Verification items for the finished model (mm, model axes). Round coordinates to 2 decimals unless told otherwise and drop trailing zeros. Order: outer loops, then holes, each group sorted by start corner. A loop starts at its lowest first (then second) coordinate and runs counter-clockwise, first axis right, second up. Notation, with made-up numbers: M 27,16.25 L 57,16.25 A19 ccw 57,31.25 Z; hole C 71,-25.5 d2. An arc over 180 degrees is marked long. Use one line per item in the form item = value. Start each with the question number.
Item 1: Go/stop test with flat-tipped pins: pin 1 Ø1.5 at (y, z) = (21, 1.5) entering from -X; pin 2 Ø3 at (y, z) = (-32.5, 1) entering from +X. Record where each tip stops, or that it passes through.
Item 2: Cross-section at A-A on x = 31.5. Enter the section's corners in (y, z).
Item 3: Cross-section at B-B on y = 22. Enter the section's corners in (x, z), then the cut area to 3 significant figures.
Item 4: Thickness scan on probe 1 along X at (y, z) = (-24, 4.75); probe 2 along X at (y, z) = (12.5, 1.8); probe 3 along Y at (x, z) = (-186, 1.5). Record the ranges inside material, lowest first. Write a range as [from, to].
Item 5: Cross-section at C-C on z = 2.9. Count the separate pieces of the cut face and the enclosed holes in it, then the cut area to 3 significant figures.
from build123d import *

# Parameters (mm, degrees)
SKETCH1_W           = 452
SKETCH1_H           = 90
BOSS_EXTRUDE1_DEPTH = 5
SKETCH2_W           = 5.2
SKETCH2_H           = 25.2
CUT_EXTRUDE1_DEPTH  = 231.490780727
SKETCH4_W           = 5
SKETCH4_H           = 30
CUT_EXTRUDE5_DEPTH  = 5
SKETCH7_R           = 1
CUT_EXTRUDE6_DEPTH  = 231.490780727
FILLET4_R           = 1
SKETCH8_W           = 20.2
SKETCH8_H           = 10
CUT_EXTRUDE7_DEPTH  = 10
SKETCH9_W           = 20.2
SKETCH9_H           = 10
CUT_EXTRUDE8_DEPTH  = 300


with BuildPart() as part:
    # Sketch1 → Boss-Extrude1 (new body)
    with BuildSketch(Plane.XY):
        Rectangle(SKETCH1_W, SKETCH1_H)
    extrude(amount=BOSS_EXTRUDE1_DEPTH)

    # Sketch2 → Cut-Extrude1 (cut, through all)
    with BuildSketch(Plane.XY.offset(5)):
        with Locations((0, 17.4)):
            Rectangle(SKETCH2_W, SKETCH2_H)
        with Locations((0, -17.4)):
            Rectangle(SKETCH2_W, SKETCH2_H)
    extrude(amount=-CUT_EXTRUDE1_DEPTH, mode=Mode.SUBTRACT)

    # Sketch4 → Cut-Extrude5 (cut)
    with BuildSketch(Plane.ZY.offset(226)):
        with Locations((2.5, 25)):
            Rectangle(SKETCH4_W, SKETCH4_H)
        with Locations((2.5, -25)):
            Rectangle(SKETCH4_W, SKETCH4_H)
    cut_extrude5 = extrude(amount=-CUT_EXTRUDE5_DEPTH, mode=Mode.SUBTRACT)

    # Mirror2: Cut-Extrude5 across plane
    add(cut_extrude5.mirror(Plane(origin=(0, 0, 0), x_dir=(0, 0, 1), z_dir=(1, 0, 0))), mode=Mode.SUBTRACT)

    # Sketch7 → Cut-Extrude6 (cut, through all)
    with BuildSketch(Plane.XY.offset(5)):
        with Locations((-221, 39)):
            Circle(SKETCH7_R)
        with Locations((-221, 11)):
            Circle(SKETCH7_R)
        with Locations((-221, -11)):
            Circle(SKETCH7_R)
        with Locations((-221, -39)):
            Circle(SKETCH7_R)
        with Locations((221, -39)):
            Circle(SKETCH7_R)
        with Locations((221, -11)):
            Circle(SKETCH7_R)
        with Locations((221, 11)):
            Circle(SKETCH7_R)
        with Locations((221, 39)):
            Circle(SKETCH7_R)
    extrude(amount=-CUT_EXTRUDE6_DEPTH, mode=Mode.SUBTRACT)

    # Fillet4
    fillet4_edges = [part.edges().sort_by_distance(p)[0] for p in [
        (221, 38, 2.5),
        (221, 12, 2.5),
        (221, -12, 2.5),
        (221, -38, 2.5),
        (-221, 38, 2.5),
        (-221, 12, 2.5),
        (-221, -38, 2.5),
        (-221, -12, 2.5),
        (-226, 10, 2.5),
        (-226, 40, 2.5),
        (-226, -40, 2.5),
        (-226, -10, 2.5),
        (226, 10, 2.5),
        (226, 40, 2.5),
        (226, -40, 2.5),
        (226, -10, 2.5),
    ]]
    fillet(fillet4_edges, radius=FILLET4_R)

    # Sketch8 → Cut-Extrude7 (cut)
    with BuildSketch(Plane(origin=(0, -610.456150304, 0), x_dir=(-1, 0, 0), z_dir=(0, 0, -1))):
        with Locations((-196, 585.456150304)):
            Rectangle(SKETCH8_W, SKETCH8_H)
    cut_extrude7 = extrude(amount=-CUT_EXTRUDE7_DEPTH, mode=Mode.SUBTRACT)

    # Mirror3: Cut-Extrude7 across plane
    add(cut_extrude7.mirror(Plane(origin=(0, 0, 0), x_dir=(0, 0, 1), z_dir=(1, 0, 0))), mode=Mode.SUBTRACT)

    # Sketch9 → Cut-Extrude8 (cut)
    with BuildSketch(Plane(origin=(0, -610.456150304, -223.6), x_dir=(-1, 0, 0), z_dir=(0, 0, -1))):
        with Locations((27.5, 585.456150304)):
            Rectangle(SKETCH9_W, SKETCH9_H)
    cut_extrude8 = extrude(amount=-CUT_EXTRUDE8_DEPTH, mode=Mode.SUBTRACT)

    # Mirror4: Cut-Extrude8 across plane
    add(cut_extrude8.mirror(Plane(origin=(0, 0, 0), x_dir=(0, 0, 1), z_dir=(1, 0, 0))), mode=Mode.SUBTRACT)


solid = part.part
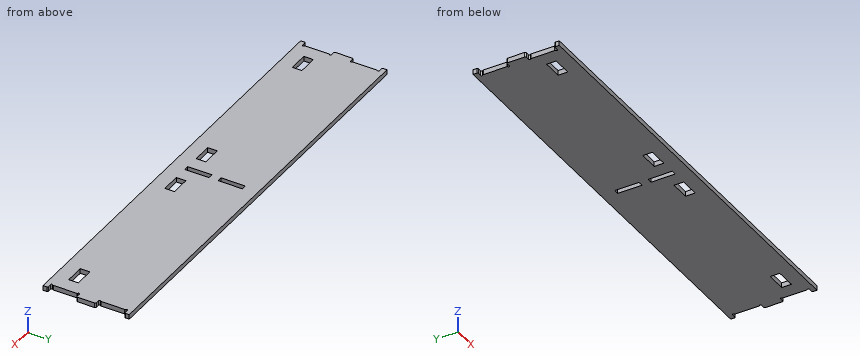
Output values:
q1.pin_1 = -221
q1.pin_2 = 221
q2.outline = M -45,0 L -30,0 L -30,5 L -45,5 Z; M -20,0 L 45,0 L 45,5 L -20,5 Z
q3.outline = M -221,0 L -2.6,0 L -2.6,5 L -221,5 Z; M 2.6,0 L 221,0 L 221,5 L 2.6,5 Z
q3.area = 2,180 mm2
q4.probe_1 = [-221, -206.1], [-185.9, -37.6], [-17.4, -2.6], [2.6, 17.4], [37.6, 185.9], [206.1, 221]
q4.probe_2 = [-220.97, -2.6], [2.6, 220.97]
q4.probe_3 = [-45, -30], [-20, 45]
q5.separate_pieces = 1
q5.enclosed_holes = 6
q5.area = 39,000 mm2
